from build123d import *

# Parameters (mm, degrees)
F2_R        = 1.5
F3_SIZE     = 1.5
F4_S7_R     = 4
F4_T8_DEPTH = 9


# Not quite as in the source:
# - a fillet or chamfer that OpenCascade refuses, or shapes differently, is made with other operations: its cross-section is extruded or revolved along the edge and cut away or added


with BuildPart() as f1:
    # F0 (on Front) → F1 (revolve)
    with BuildSketch(Plane.XZ):
        Polygon((0, 130), (0, 0), (25, 0), (25, 5), (10, 5), (10, 90), (4, 90), (4, 91.8505489826), (5, 91.8505489826), (5, 130), align=None)
    revolve(axis=Axis((0, 0, 65), (0, 0, 1)))

    # F2
    f2_edges = [f1.edges().sort_by_distance(p)[0] for p in [
        (-10, 0, 5),
    ]]
    fillet(f2_edges, radius=F2_R)

    # F3
    f3_edges = [f1.edges().sort_by_distance(p)[0] for p in [
        (-25, 0, 5),
        (-25, 0, 0),
    ]]
    chamfer(f3_edges, length=F3_SIZE)

    # F4: chamfer of 1.6 on 2 edges, made by hand

    # F4_s1 → F4_t2 (revolve, cut)
    with BuildSketch(Plane.XZ):
        Polygon((5, 128.4), (3.4, 130), (5, 130), align=None)
    revolve(axis=Axis((0, 0, 130), (0, 0, 1)), mode=Mode.SUBTRACT)


with BuildPart() as f4_tool4:
    # F4_s5 → F4_t6 (revolve)
    with BuildSketch(Plane.XZ):
        Polygon((3.4, 91.8505489826), (5, 93.4505489826), (5, 91.8505489826), align=None)
    revolve(axis=Axis((0, 0, 91.8505489826), (0, 0, 1)))

    # F4_s7 → F4_t8 (cut, symmetric)
    with BuildSketch(Plane.XY.offset(92.7)):
        Circle(F4_S7_R)
    extrude(amount=F4_T8_DEPTH, both=True, mode=Mode.SUBTRACT)


with BuildPart() as f1_1:
    add(f1.part)

    # F4_t3: cut F4_tool4
    add(f4_tool4.part, mode=Mode.SUBTRACT)


solid = f1_1.part
Input: part model. Units: mm. Frame: model coordinates. A direction names the side the tool comes from. Round coordinates to 2 decimals unless told otherwise and drop trailing zeros. Write each loop counter-clockwise with the first axis right and the second up, starting at its lowest first coordinate (ties: lowest second). Pieces come first, ordered by that corner, then holes.
1) Cut plane C-C (z = 97.5). Return the cut outline in (x, y).
2) Cut plane A-A (x = 0). Return the cut outline in (y, z), then the cut area to 3 significant figures.
3) Draft query along Z for faces 4 (the flat face through (0, 0, 130)), 5 (the flat face through (0, 0, 0)), 6 (the cylindrical face through (-1.08, -4.88, 111.17)), 7 (the cylindrical face through (-0.867, -3.905, 91.242)). Return one class per face: pulls with the +Z half, pulls with the -Z half, needs draft (parallel to the pull), parting line crosses it, or undercut.
4) Cut plane D-D (z = 78). Return the cut outline in (x, y).
5) Ray query, L1, parallel to Z at x = 13.5, y = 11.5; L2, parallel to Z at x = -5, y = 5.5; L3, parallel to Y at x = 0.5, z = 80. Return the intervals inside material, ascending.
6) Contact query for flat-ended pins moving along their axis: P1, Ø8, axis at x = 11, z = 61.5, coming from the -Y side; P2, Ø5, axis at x = -13, y = 15, coming from the +Z side; P3, Ø10, axis at x = 6.5, y = -0.5, coming from the +Z side; P4, Ø6, axis at y = -8, z = 60, coming from the +X side. Output: stop coordinate, or through.
7) Reachability of faces 1 (the cylindrical face through (-2.17, -9.76, 48.83)), 2 (the flat face through (4.3, 0.1, 90)), 3 (the cylindrical face through (23.846, 7.509, 2.514)) from +Z, -Z, +X, -X, +Y, -Y: full face, straight path, thin tool, end or side. Return the list, or none.
Geometry says:
1. outline: circle Ø10 at (0, 0)
2. outline: (-25, 1.5) - (-23.5, 0) - (23.5, 0) - (25, 1.5) - (25, 3.5) - (23.5, 5) - (11.5, 5) arc R1.5 cw to (10, 6.5) - (10, 90) - (4, 90) - (4, 92.45) - (5, 93.45) - (5, 128.4) - (3.4, 130) - (-3.4, 130) - (-5, 128.4) - (-5, 93.45) - (-4, 92.45) - (-4, 90) - (-10, 90) - (-10, 6.5) arc R1.5 cw to (-11.5, 5) - (-23.5, 5) - (-25, 3.5) - close
2. area: 2,340 mm2
3. face 4: pulls with the +Z half
3. face 5: pulls with the -Z half
3. face 6: needs draft
3. face 7: undercut
4. outline: circle Ø20 at (0, 0)
5. L1: z = 0 to 5
5. L2: z = 0 to 90
5. L3: y = -9.99 to 9.99
6. P1: stops at y = -7.14
6. P2: stops at z = 5
6. P3: stops at z = 130
6. P4: stops at x = 8.66
7. face 1: +Z
7. face 2: none
7. face 3: +Z, -Z
